Source: CAD feature listing. Evaluate the final solid. Frame: model axes, mm. A direction names the side the tool comes from. Coordinates: 2 decimals unless noted, no trailing zeros. Loops run counter-clockwise (first coordinate to the right, second up) from the corner with the lowest first, then second, coordinate; pieces in that order, holes last.
Item 1: Section query B-B, the plane y = -25. Return the cut outline in (x, z), then the cut area to 3 significant figures.
Item 2: Section query C-C, the plane z = 12.6. State how many separate pieces and enclosed holes the cut face has, then the cut area to 3 significant figures.
Item 3: Pull-direction query (X, two-part tool) for faces 1 (the flat face through (72, -66, 14)), 2 (the flat face through (0.21, 25.4, 13.96)), 3 (the flat face through (78.8, -70, 14)); classes: +X half, -X half, draft (parallel to the pull), parting line (faces both ways), or undercut.
Item 4: Pin query (flat end, axial travel): pin 1 Ø2 at (x, z) = (-32, 13) entering from -Y; pin 2 Ø2.5 at (x, z) = (-74, 13) entering from +Y; pin 3 Ø1.8 at (x, y) = (-82.3, -19.8) entering from +Z; pin 4 Ø1 at (y, z) = (30, 12) entering from +X. Return the tip coordinate at first contact, or that it passes through.
Item 5: Section query A-A, the plane x = -27. Return the cut outline in (y, z).
Item 6: Reachability of faces 4 (the flat face through (13, -40, 11)), 5 (the flat face through (-50, 22.5, 14)), 6 (the flat face through (-16.2, -9, 13)) from +Z, -Z, +X, -X, +Y, -Y: full face, straight path, thin tool, end or side. Return the list, or none.
Item 7: Line query: probe 1 along Y at (x, z) = (-17.7, 16.25); probe 2 along X at (y, z) = (-19.8, 16.15); probe 3 along Y at (x, z) = (-39, 14.8). Output: solid intervals per line, ascending.
```python
from build123d import *

# Parameters (mm, degrees)
PAD001_DEPTH    = 6
THICKNESS001_T  = -1.2
SKETCH011_R     = 1.5
POCKET003_DEPTH = 1.2
SKETCH012_W     = 15
SKETCH012_H     = 15
POCKET004_DEPTH = 6.001
SKETCH013_R     = 2.6
POCKET005_DEPTH = 1.2
SKETCH014_R     = 2.6
POCKET006_DEPTH = 1.2
SKETCH015_R     = 2.6
POCKET007_DEPTH = 1.2


with BuildPart() as part:
    # Sketch004 → Pad001 (new body)
    with BuildSketch(Plane.XY):
        Polygon((80, -74), (65, -74), (-15, -22.5), (-85, -22.5), (-85, 22.5), (-15, 22.5), (15, 44), (30, 44), (30, 36), (15, 36), (-15, 14.5), (-15, 4), (0, 4), (0, -4), (-15, -4), (-15, -14.5), (65, -66), (80, -66), align=None)
    extrude(amount=PAD001_DEPTH)

    # Thickness001
    thickness001_openings = [part.faces().sort_by_distance(p)[0] for p in [
        (-29.840547, -5.671982, 0),
    ]]
    offset(amount=THICKNESS001_T, openings=thickness001_openings, kind=Kind.INTERSECTION)

    # Sketch011 (on Face19 of Thickness001) → Pocket003 (cut)
    with BuildSketch(Plane.XY.offset(6)):
        with Locations((-82.3, 19.8)):
            Circle(SKETCH011_R)
        with Locations((-82.3, -19.8)):
            Circle(SKETCH011_R)
        with Locations((-17.7, 11.8)):
            Circle(SKETCH011_R)
        with Locations((-17.7, -11.8)):
            Circle(SKETCH011_R)
    extrude(amount=-POCKET003_DEPTH, mode=Mode.SUBTRACT)

    # Sketch012 (on Face5 of Pocket003) → Pocket004 (cut, through all)
    with BuildSketch(Plane.XY.offset(6)):
        with Locations((-62.5, -15)):
            Rectangle(SKETCH012_W, SKETCH012_H)
    extrude(amount=-POCKET004_DEPTH, mode=Mode.SUBTRACT)

    # Sketch013 (on Face16 of Pocket004) → Pocket005 (cut)
    with BuildSketch(Plane.YZ.offset(30)):
        with Locations((40, 0)):
            Circle(SKETCH013_R)
    extrude(amount=-POCKET005_DEPTH, mode=Mode.SUBTRACT)

    # Sketch014 (on Face11 of Pocket005) → Pocket006 (cut)
    with BuildSketch(Plane.YZ):
        Circle(SKETCH014_R)
    extrude(amount=-POCKET006_DEPTH, mode=Mode.SUBTRACT)

    # Sketch015 (on Face2 of Pocket006) → Pocket007 (cut)
    with BuildSketch(Plane.YZ.offset(80)):
        with Locations((-70, 0)):
            Circle(SKETCH015_R)
    extrude(amount=-POCKET007_DEPTH, mode=Mode.SUBTRACT)


with BuildPart() as part_1:
    # Body001 placement: moved
    add(part.part.moved(Location((0, 0, 11))))


solid = part_1.part
```
Verdict:
1. outline: (-11.12, 11) - (-8.9, 11) - (-8.9, 15.8) - (-0.91, 15.8) - (-0.91, 11) - (1.31, 11) - (1.31, 17) - (-11.12, 17) - close
1. area: 36.2 mm2
2. separate pieces: 4
2. enclosed holes: 0
2. area: 662 mm2
3. face 1: draft
3. face 2: +X half
3. face 3: undercut
4. pin 1: stops at y = -22.5
4. pin 2: stops at y = 22.5
4. pin 3: passes through
4. pin 4: stops at x = 7.33
5. outline: (-22.5, 11) - (-21.3, 11) - (-21.3, 15.8) - (21.3, 15.8) - (21.3, 11) - (22.5, 11) - (22.5, 17) - (-22.5, 17) - close
6. face 4: -Z, +X, -X, +Y, -Y
6. face 5: +Z, -Z, -X, +Y
6. face 6: -Z
7. probe 1: y = -22.5 to -13.3, -10.3 to 10.3, 13.3 to 22.5
7. probe 2: x = -85 to -83.8, -80.8 to -70, -55 to -6.77
7. probe 3: y = -22.5 to -21.3, 21.3 to 22.5
